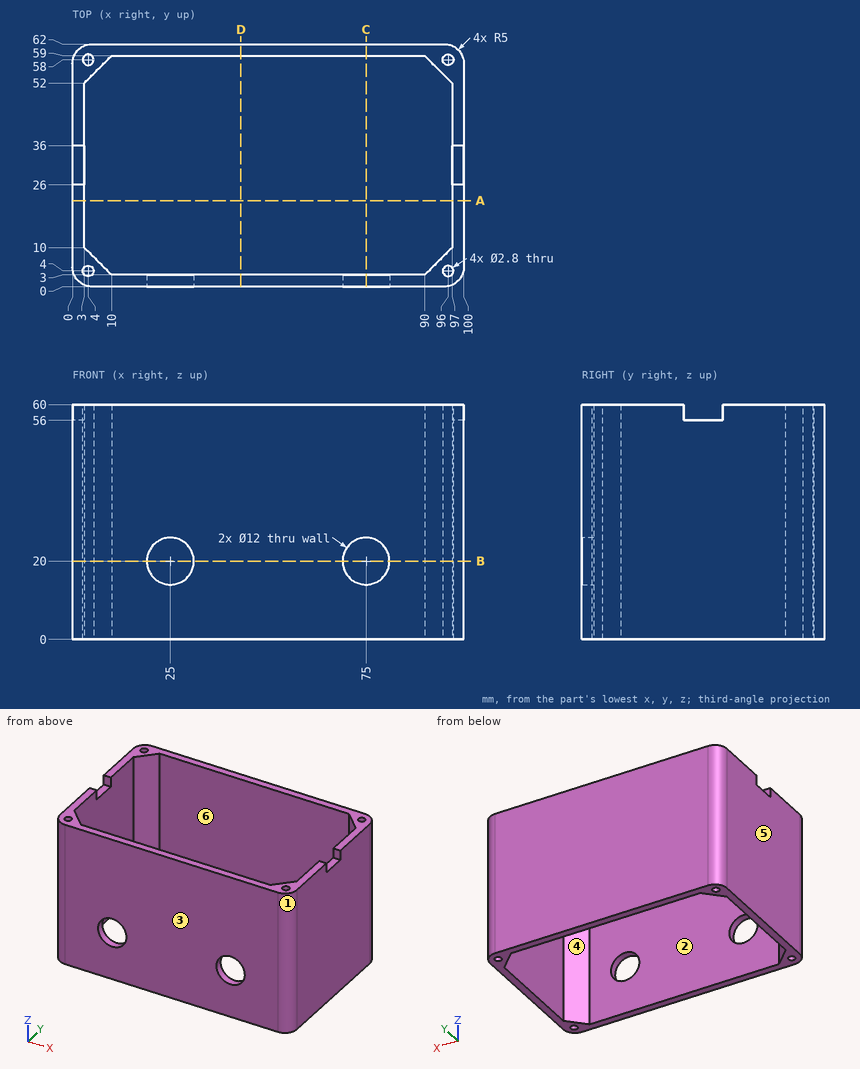
The figure shows three views and two pictorial views of one solid part (mm, origin at its lowest corner). Answer the questions. A direction names the side the tool comes from. Round coordinates to 2 decimals unless told otherwise and drop trailing zeros. Write each loop counter-clockwise with the first axis right and the second up, starting at its lowest first coordinate (ties: lowest second). Pieces come first, ordered by that corner, then holes. Notation, with made-up numbers: (18.5, 58.25) - (60.5, 58.25) arc R21 ccw to (60.5, 85.25) - close; hole circle Ø5 at (-26.5, -4). An arc over 180 degrees is marked (long way). Answer in a Markdown table with one row per item. Add a question column.
1. The mould has two halves that part along X. Classify the marked faces 1, 2, 3 and 4: +X half, -X half, draft (parallel to the pull), parting line (faces both ways), or undercut.
2. Find the intervals of material crossed by line 1 along Y through (x, z) = (67.5, 25); line 2 along X through (y, z) = (11.5, 17.5); line 3 along X through (y, z) = (4, 38), in increasing order. Write a range as from..to.
3. Given pin 1 (2 mm diameter, centred on x = 4, y = 58, fed in from -Z); pin 2 (2 mm diameter, centred on y = 35.5, z = 34, fed in from -X); pin 3 (0.9 mm diameter, centred on x = 1, z = 57.5, fed in from -Y); pin 4 (1.5 mm diameter, centred on x = 98, z = 58.5, fed in from +Y), each flat-ended and moving along its own axis, determine where each tip first touches the part or whether it passes through.
4. For the marked faces 5 and 6, determine the directions among +Z, -Z, +X, -X, +Y, -Y from which every point of the face is accessible in a straight line to the end or side of a thin tool.
5. A cutting plane is placed at B-B, the plane z = 20. Determine the outline of the cut face in (x, y).
6. A cutting plane is placed at D-D, the plane x = 43. Determine the outline of the cut face in (y, z).
7. A cutting plane is placed at A-A, the plane y = 22. Determine the outline of the cut face in (x, z), and give its area (3 significant figures).
8. A cutting plane is placed at C-C, the plane x = 75. Determine the outline of the cut face in (y, z).
Worked out:
| question | item | result |
|---|---|---|
| 1 | face 1 | +X half |
| 1 | face 2 | undercut |
| 1 | face 3 | draft |
| 1 | face 4 | undercut |
| 2 | line 1 | 0..3, 59..62 |
| 2 | line 2 | 0..3, 97..100 |
| 2 | line 3 | 0.1..2.6, 5.4..9, 91..94.6, 97.4..99.9 |
| 3 | pin 1 | through |
| 3 | pin 2 | x = 0 |
| 3 | pin 3 | y = 1.48 |
| 3 | pin 4 | y = 61.47 |
| 4 | face 5 | +Z, -Z, -X, +Y, -Y |
| 4 | face 6 | +Z, -Z |
| 5 | outline | (0, 5) arc R5 ccw to (5, 0) - (19, 0) - (19, 3) - (10, 3) - (3, 10) - (3, 52) - (10, 59) - (90, 59) - (97, 52) - (97, 10) - (90, 3) - (81, 3) - (81, 0) - (95, 0) arc R5 ccw to (100, 5) - (100, 57) arc R5 ccw to (95, 62) - (5, 62) arc R5 ccw to (0, 57) - close; (31, 0) - (69, 0) - (69, 3) - (31, 3) - close; hole circle Ø2.8 at (4, 4); hole circle Ø2.8 at (4, 58); hole circle Ø2.8 at (96, 4); hole circle Ø2.8 at (96, 58) |
| 6 | outline | (0, 0) - (3, 0) - (3, 60) - (0, 60) - close; (59, 0) - (62, 0) - (62, 60) - (59, 60) - close |
| 7 | outline | (0, 0) - (3, 0) - (3, 60) - (0, 60) - close; (97, 0) - (100, 0) - (100, 60) - (97, 60) - close |
| 7 | area | 360 mm^2 |
| 8 | outline | (0, 0) - (3, 0) - (3, 14) - (0, 14) - close; (0, 26) - (3, 26) - (3, 60) - (0, 60) - close; (59, 0) - (62, 0) - (62, 60) - (59, 60) - close |
